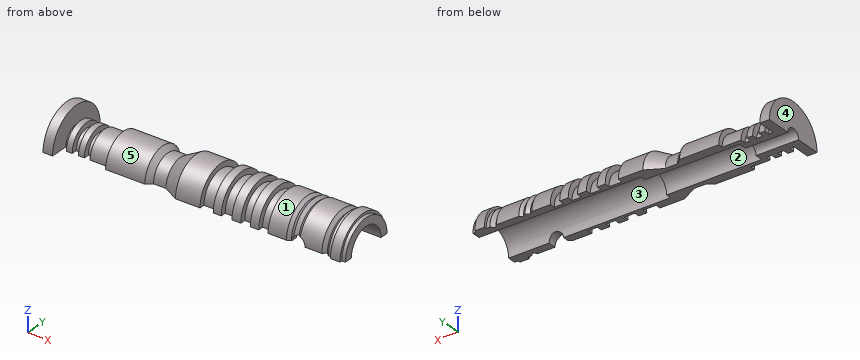
from build123d import *

# Parameters (mm, degrees)
F1_ANGLE = -180
F2_R     = 4.5
F3_DEPTH = 127.6
F4_R     = 12.5
F5_DEPTH = 100
F6_R     = 4.5
F7_DEPTH = 16.8
F8_R     = 9.247481
F9_DEPTH = 58.7


with BuildPart() as f1:
    # F0 (on Top) → F1 (revolve)
    with BuildSketch(Plane.XY):
        Polygon((-150, 5), (-125.782207, 5), (-122.500561, 7.857719), (-114.843413, 7.857719), (-105, 2.5), (-89.808904, 2.5), (-89.808904, 5.75), (-81.664719, 5.75), (-81.664719, 2.5), (-76.673128, 2.5), (-76.673128, 5.75), (-70.105232, 5.75), (-70.105232, 2.5), (-64.588204, 2.5), (-64.588204, 5.75), (-58.808461, 5.75), (-58.808461, 2.5), (-53.554147, 2.5), (-53.554147, 5.75), (-47.774404, 5.75), (-47.774404, 2.5), (-36.38434, 2.5), (-34.337129, 3.887209), (-32.161966, 2.5), (-30.114755, 3.887209), (-28.323445, 2.5), (-14.525713, 2.5), (-12.570513, 4.523719), (-10.475874, 2.5), (-8.125912, 2.5), (-8.125912, 1.010104), (-2.228058, 1.010104), (-2.228058, 2.5), (0, 2.5), (0, 20), (-185, 20), (-185, 0), (-179.089636, 0), (-179.089636, 11.18013), (-176.320955, 11.18013), (-176.320955, 7.857719), (-172.721684, 7.857719), (-172.721684, 11.18013), (-168.845534, 11.18013), (-168.845534, 7.857719), (-165.246248, 7.857719), (-165.246248, 11.18013), (-161.646977, 11.18013), (-161.646977, 7.857719), (-150, 7.857719), align=None)
    revolve(axis=Axis((-92.5, 20, 0), (1, 0, 0)), revolution_arc=F1_ANGLE)

    # F2 (on face) → F3 (cut)
    with BuildSketch(Plane(origin=(-185, 0, 0), x_dir=(0, -1, 0), z_dir=(-1, 0, 0))):
        with Locations((-20, 0)):
            Circle(F2_R)
    extrude(amount=-F3_DEPTH, mode=Mode.SUBTRACT)

    # F4 (on face) → F5 (cut)
    with BuildSketch(Plane.YZ):
        with Locations((20, 0)):
            Circle(F4_R)
    extrude(amount=-F5_DEPTH, mode=Mode.SUBTRACT)

    # F6 (on Front) → F7 (cut)
    with BuildSketch(Plane.XZ):
        with Locations((-29.463233, 0)):
            Circle(F6_R)
    extrude(amount=-F7_DEPTH, mode=Mode.SUBTRACT)

    # F8 (on face) → F9 (cut)
    with BuildSketch(Plane.YZ.offset(-100)):
        with Locations((20, 0)):
            Circle(F8_R)
    extrude(amount=-F9_DEPTH, mode=Mode.SUBTRACT)


solid = f1.part
Build history of the part. All positions in model axes, mm. Face numbers are marked on the shaded views. A direction names the side the tool comes from. Coordinates: 2 decimals unless noted, no trailing zeros. Write each loop counter-clockwise with the first axis right and the second up, starting at its lowest first coordinate (ties: lowest second). Pieces come first, ordered by that corner, then holes.
(1) Cut at A-A on x = -130.5. List the corners of the cut face in (y, z), and give its area (3 significant figures).
(2) Pin check, flat tips, straight feed: pin 1 Ø4 at (y, z) = (24, 9) entering from +X; pin 2 Ø12 at (x, z) = (-115.5, 3) entering from -Y; pin 3 Ø12 at (x, z) = (-110, 10.5) entering from -Y; pin 4 Ø1.5 at (x, z) = (-49.5, 17.5) entering from -Y. Stop position of each tip, or through.
(3) Mould opens along Y. For the marked faces 3, 4 and 5 say: pulls with the +Y half, pulls with the -Y half, needs draft (parallel to the pull), parting line crosses it, or undercut.
(4) Drill centre lines: line 1 (X direction, y = 10, z = 4.25); line 2 (X direction, y = 7.5, z = 12.75); line 3 (X direction, y = 25.5, z = 12.5). Where is each one in solid material? Low to high.
(5) 3-axis set-ups, long thin cutter, end or side, ignore diameter. For the marked faces 1 and 2: which of +Z, -Z, +X, -X, +Y, -Y reach the whole face in a straight line?
(6) Cut at B-B on x = -67.5. List the corners of the cut face in (y, z).
Working result:
1. outline: (5, 0) - (10.75, 0) arc R9.25 cw to (29.25, 0) - (35, 0) arc R15 ccw to start
1. area: 219 mm2
2. pin 1: stops at x = -100
2. pin 2: stops at y = 5.12
2. pin 3: stops at y = 4.04
2. pin 4: passes through
3. face 3: undercut
3. face 4: needs draft
3. face 5: parting line crosses it
4. line 1: x = -185 to -179.09, -176.32 to -172.72, -168.85 to -165.25, -161.65 to -100
4. line 2: x = -185 to -179.09, -8.13 to -2.23
4. line 3: x = -185 to -179.09, -150 to -124.24, -112.06 to 0
5. face 1: +Z
5. face 2: -Z, +X
6. outline: (2.5, 0) - (7.5, 0) arc R12.5 cw to (32.5, 0) - (37.5, 0) arc R17.5 ccw to start
